Input: part model. Units: mm. Frame: model coordinates. Face numbers are marked on the shaded views. A direction names the side the tool comes from. Round coordinates to 2 decimals unless told otherwise and drop trailing zeros. Loops run counter-clockwise (first coordinate to the right, second up) from the corner with the lowest first, then second, coordinate; pieces in that order, holes last.
(1) Cut plane C-C, the plane z = 4.3. Output: boundary loops of the cut face in (x, y).
(2) Access query for the marked faces 5, 6 and 7. Directions: +Z, -Z, +X, -X, +Y, -Y. A direction counts if a zero-diameter tool reaches every point of the face in a straight line with its end or side. Return the directions, or none.
(3) Draft query along Y for the marked faces 1, 2, 3 and 4. Return one class per face: released by +Y, released by -Y, zero draft, split by the parting line, or undercut.
(4) Cut plane D-D, the plane z = 0.85. Output: boundary loops of the cut face in (x, y), and give its area (3 significant figures).
(5) Cut plane A-A, the plane y = 14. Output: boundary loops of the cut face in (x, z).
(6) First-contact query: pin 1 Ø1 at (x, z) = (-5.5, 0.5) entering from -Y; pin 2 Ø2 at (y, z) = (8.5, 4) entering from -X; pin 3 Ø5.5 at (x, y) = (-4.5, 6) entering from +Z; pin 4 Ø5.5 at (x, y) = (28, 7.5) entering from +Z. Flat tips, straight axial feed; report the tip coordinate or a pass-through.
(7) Cut plane B-B, the plane x = 20. Output: boundary loops of the cut face in (y, z).
(8) Line query: line 1 (Y direction, x = 7, z = 0.3); line 2 (X direction, y = 5.25, z = 3.85); line 3 (Y direction, x = 28, z = 1.6). Output: solid intervals per line, ascending.
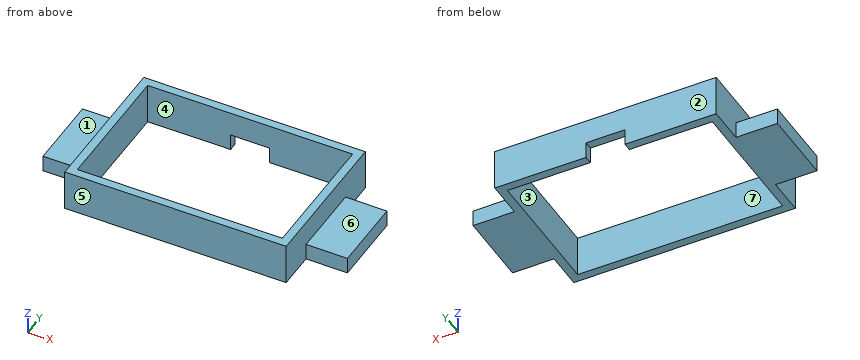
from build123d import *

# Parameters (mm, degrees)
F0_W     = 3
F0_H     = 5
F0_W_2   = 1
F0_H_2   = 1
F1_DEPTH = 2
F0_W_3   = 4.7
F2_DEPTH = 5
F3_DEPTH = 2


with BuildPart() as f1:
    # F0 (on Top) → F1 (new body)
    with BuildSketch(Plane.XY):
        with Locations((26.2, 7)):
            Rectangle(F0_W, F0_H)
        Polygon((-2, 10.5), (-1, 10.5), (-1, 15), (9, 15), (9, 16), (-2, 16), (-2, 11.5), align=None)
        with Locations((-3.5, 7)):
            Rectangle(F0_W, F0_H)
        Polygon((-2, 3.5), (-2, 4.5), (-5, 4.5), (-5, 9.5), (-2, 9.5), (-2, 10.5), (-6, 10.5), (-6, 3.5), align=None)
        Polygon((27.7, 4.5), (24.7, 4.5), (24.7, 3.5), (28.7, 3.5), (28.7, 10.5), (24.7, 10.5), (24.7, 9.5), (27.7, 9.5), align=None)
        Polygon((-2, 2.5), (-2, 3.5), (-6, 3.5), (-6, 10.5), (-2, 10.5), (-2, 11.5), (-7, 11.5), (-7, 2.5), align=None)
        Polygon((-1, -1), (-1, 3.5), (-2, 3.5), (-2, 2.5), (-2, -2), (24.7, -2), (24.7, 2.5), (24.7, 3.5), (23.7, 3.5), (23.7, -1), align=None)
        with Locations((-1.5, 7)):
            Rectangle(F0_W_2, F0_H)
        with Locations((-1.5, 4)):
            Rectangle(F0_W_2, F0_H_2)
        with Locations((24.2, 4)):
            Rectangle(F0_W_2, F0_H_2)
        with Locations((24.2, 7)):
            Rectangle(F0_W_2, F0_H)
        with Locations((24.2, 10)):
            Rectangle(F0_W_2, F0_H_2)
        Polygon((23.7, 15), (23.7, 10.5), (24.7, 10.5), (24.7, 11.5), (24.7, 16), (13.7, 16), (13.7, 15), align=None)
        Polygon((28.7, 3.5), (24.7, 3.5), (24.7, 2.5), (29.7, 2.5), (29.7, 11.5), (24.7, 11.5), (24.7, 10.5), (28.7, 10.5), align=None)
        with Locations((-1.5, 10)):
            Rectangle(F0_W_2, F0_H_2)
    extrude(amount=F1_DEPTH)

    # F0 (on Top) → F2 (join)
    with BuildSketch(Plane.XY):
        Polygon((-2, 10.5), (-1, 10.5), (-1, 15), (9, 15), (9, 16), (-2, 16), (-2, 11.5), align=None)
        with Locations((11.35, 15.5)):
            Rectangle(F0_W_3, F0_H_2)
        Polygon((23.7, 15), (23.7, 10.5), (24.7, 10.5), (24.7, 11.5), (24.7, 16), (13.7, 16), (13.7, 15), align=None)
        with Locations((24.2, 10)):
            Rectangle(F0_W_2, F0_H_2)
        with Locations((24.2, 7)):
            Rectangle(F0_W_2, F0_H)
        Polygon((-1, -1), (-1, 3.5), (-2, 3.5), (-2, 2.5), (-2, -2), (24.7, -2), (24.7, 2.5), (24.7, 3.5), (23.7, 3.5), (23.7, -1), align=None)
        with Locations((24.2, 4)):
            Rectangle(F0_W_2, F0_H_2)
        with Locations((-1.5, 4)):
            Rectangle(F0_W_2, F0_H_2)
        with Locations((-1.5, 7)):
            Rectangle(F0_W_2, F0_H)
        with Locations((-1.5, 10)):
            Rectangle(F0_W_2, F0_H_2)
    extrude(amount=F2_DEPTH)

    # F0 (on Top) → F3 (cut)
    with BuildSketch(Plane.XY):
        with Locations((11.35, 15.5)):
            Rectangle(F0_W_3, F0_H_2)
    extrude(amount=F3_DEPTH, mode=Mode.SUBTRACT)


solid = f1.part
Reported:
1. outline: (-2, -2) - (24.7, -2) - (24.7, 16) - (-2, 16) - close; hole (-1, -1) - (23.7, -1) - (23.7, 15) - (-1, 15) - close
2. face 5: +Z, -Z, +X, -X, -Y
2. face 6: +Z, +X, +Y, -Y
2. face 7: +Z, -Z
3. face 1: zero draft
3. face 2: released by +Y
3. face 3: undercut
3. face 4: undercut
4. outline: (-7, 2.5) - (-2, 2.5) - (-2, -2) - (24.7, -2) - (24.7, 2.5) - (29.7, 2.5) - (29.7, 11.5) - (24.7, 11.5) - (24.7, 16) - (13.7, 16) - (13.7, 15) - (23.7, 15) - (23.7, -1) - (-1, -1) - (-1, 15) - (9, 15) - (9, 16) - (-2, 16) - (-2, 11.5) - (-7, 11.5) - close
4. area: 171 mm2
5. outline: (-2, 0) - (-1, 0) - (-1, 5) - (-2, 5) - close; (23.7, 0) - (24.7, 0) - (24.7, 5) - (23.7, 5) - close
6. pin 1: stops at y = 2.5
6. pin 2: stops at x = -2
6. pin 3: stops at z = 5
6. pin 4: stops at z = 2
7. outline: (-2, 0) - (-1, 0) - (-1, 5) - (-2, 5) - close; (15, 0) - (16, 0) - (16, 5) - (15, 5) - close
8. line 1: y = -2 to -1, 15 to 16
8. line 2: x = -2 to -1, 23.7 to 24.7
8. line 3: y = 2.5 to 11.5
